```python
from build123d import *

# Parameters (mm, degrees)
F3_W     = 29.70758
F3_H     = 25.697972
F4_DEPTH = 25.4
F5_R     = 0.375966
F6_DEPTH = 0.254
F5_R_2   = 0.381
F7_DEPTH = 0.254


with BuildPart() as f1:
    # F0 (on Front) → F1 (revolve)
    with BuildSketch(Plane.XZ):
        with BuildLine():
            Line((0, 12.7), (0, -12.7))
            ThreePointArc((0, -12.7), (12.7, 0), (0, 12.7))
        make_face()
    revolve(axis=Axis((0, 0, 0), (0, 0, -1)))

    # F3 (on offset) → F4 (cut)
    with BuildSketch(Plane.XY):
        Rectangle(F3_W, F3_H)
    extrude(amount=-F4_DEPTH, mode=Mode.SUBTRACT)

    # F5 (on Top) → F6 (cut)
    with BuildSketch(Plane.XY):
        Circle(F5_R)
    extrude(amount=F6_DEPTH, mode=Mode.SUBTRACT)

    # F5 (on Top) → F7 (cut)
    with BuildSketch(Plane.XY):
        Circle(F5_R)
        with Locations((0, -12.192)):
            Circle(F5_R_2)
        with Locations((0, 12.192)):
            Circle(F5_R_2)
        with Locations((12.192, 0)):
            Circle(F5_R_2)
        with Locations((-12.192, 0)):
            Circle(F5_R_2)
    extrude(amount=F7_DEPTH, mode=Mode.SUBTRACT)


solid = f1.part
```
CAD build for the part. Positions are in the model's coordinates, mm. Coordinates: 2 decimals unless noted, no trailing zeros. Order: outer loops, then holes, each group sorted by start corner. A loop starts at its lowest first (then second) coordinate and runs counter-clockwise, first axis right, second up. Notation, with made-up numbers: (34, 23) -> (56, 23) arc R17 cw to (56, 51) -> close; hole circle Ø5 at (-39, -12). An arc over 180 degrees is marked (long way). Use one line per item in the form item = value. Start each with the question number.
1) Band-saw the part on A-A on x = 0. Give the cut face in (y, z), then the cut area to 3 significant figures.
2) Drill centre lines: L1, parallel to Y at x = 2.5, z = 7.75; L2, parallel to X at y = -10.5, z = 4.75; L3, parallel to Z at x = 2.5, y = 0. Where is each one in solid material? Low to high. Write a range as [from, to].
3) Drop flat-ended pins along their axis: pin 1 (1.5 mm diameter, centred on y = -0.5, z = 7.5, fed in from -X); pin 2 (5 mm diameter, centred on y = 0.5, z = 4, fed in from -X); pin 3 (1 mm diameter, centred on x = -3, z = 5, fed in from -Y). Give the stop position or say it passes through.
4) Band-saw the part on D-D on z = 8.25. Give the cut face in (x, y), then the cut area to 3 significant figures.
5) Band-saw the part on C-C on z = 10. Give the cut face in (x, y).
Entries:
q1.outline = (-12.7, 0) -> (-12.57, 0) -> (-12.57, 0.25) -> (-11.81, 0.25) -> (-11.81, 0) -> (-0.38, 0) -> (-0.38, 0.25) -> (0.38, 0.25) -> (0.38, 0) -> (11.81, 0) -> (11.81, 0.25) -> (12.57, 0.25) -> (12.57, 0) -> (12.7, 0) arc R12.7 ccw to start
q1.area = 253 mm2
q2.L1 = [-9.75, 9.75]
q2.L2 = [-5.34, 5.34]
q2.L3 = [0, 12.45]
q3.pin_1 = -10.75
q3.pin_2 = -12.61
q3.pin_3 = -11.53
q4.outline = circle Ø19.31 at (0, 0)
q4.area = 293 mm2
q5.outline = circle Ø15.66 at (0, 0)
